```python
from build123d import *

# Parameters (mm, degrees)
F0_W     = 35.3
F0_H     = 35.3
F0_R     = 1.5
F1_DEPTH = 13
F2_R     = 11
F3_DEPTH = 2
F4_R     = 2.25
F5_DEPTH = 24
F7_DEPTH = 3.625
F8_SIZE  = 2.5


with BuildPart() as f1:
    # F0 (on Front) → F1 (new body, symmetric)
    with BuildSketch(Plane.XZ):
        Rectangle(F0_W, F0_H)
        with Locations((-13, -13)):
            Circle(F0_R, mode=Mode.SUBTRACT)
        with Locations((13, -13)):
            Circle(F0_R, mode=Mode.SUBTRACT)
        with Locations((-13, 13)):
            Circle(F0_R, mode=Mode.SUBTRACT)
        with Locations((13, 13)):
            Circle(F0_R, mode=Mode.SUBTRACT)
    extrude(amount=F1_DEPTH, both=True)

    # F2 (on face) → F3 (join)
    with BuildSketch(Plane.XZ.offset(13)):
        Circle(F2_R)
    extrude(amount=F3_DEPTH)

    # F4 (on face) → F5 (join)
    with BuildSketch(Plane.XZ.offset(15)):
        Circle(F4_R)
    extrude(amount=F5_DEPTH)

    # F6 (on Front) → F7 (cut, symmetric)
    with BuildSketch(Plane.XZ):
        Polygon((17.65, 17.65), (11.9931457505, 17.65), (17.65, 11.9931457505), align=None)
        Polygon((11.9931457505, -17.65), (17.65, -17.65), (17.65, -11.9931457505), align=None)
        Polygon((-17.65, -11.9931457505), (-17.65, -17.65), (-11.9931457505, -17.65), align=None)
        Polygon((-11.9931457505, 17.65), (-17.65, 17.65), (-17.65, 11.9931457505), align=None)
    extrude(amount=F7_DEPTH, both=True, mode=Mode.SUBTRACT)

    # F8
    f8_edges = [f1.edges().sort_by_distance(p)[0] for p in [
        (17.65, -8.3125, 17.65),
        (17.65, 8.3125, 17.65),
        (-17.65, 8.3125, 17.65),
        (-17.65, -8.3125, 17.65),
        (17.65, 8.3125, -17.65),
        (17.65, -8.3125, -17.65),
        (-17.65, -8.3125, -17.65),
        (-17.65, 8.3125, -17.65),
    ]]
    chamfer(f8_edges, length=F8_SIZE)


solid = f1.part
```
Source: CAD feature listing. Evaluate the final solid. Frame: model axes, mm. A direction names the side the tool comes from. Give positions to 0.01 mm unless a question says otherwise; leave off trailing zeros. Loops run counter-clockwise (first coordinate to the right, second up) from the corner with the lowest first, then second, coordinate; pieces in that order, holes last. Notation, with made-up numbers: (46, 19) -> (62, 19) arc R21 cw to (62, 23) -> close; hole circle Ø3 at (80, 9). An arc over 180 degrees is marked (long way). Put each result on its own line as item: value. Start each with the question number.
1) Cut plane B-B (x = 13). Return loops of the section in (y, z) (3 decimals), then the cut area to 3 significant figures.
2) Reachability of faces 4 (the face through (-2.38, -13.99, -10.74)), 5 (the face through (-15, 3.625, -15)), 6 (the face through (14.861, 0.051, -14.782)), 7 (the face through (-15, 3.625, 15)) from +Z, -Z, +X, -X, +Y, -Y: full face, straight path, thin tool, end or side. Return the list, or none.
3) Cut plane D-D (x = 0). Return loops of the section in (y, z).
4) Contact query for flat-ended pins moving along their axis: P1, Ø10.5, axis at x = 3, z = -2, coming from the -Y side; P2, Ø5, axis at x = -6.5, y = -31, coming from the +Z side; P3, Ø4.5, axis at x = -15, z = -15.5, coming from the -Y side; P4, Ø1, axis at x = 2.5, y = -18.5, coming from the -Z side. Output: stop coordinate, or through.
5) Material intervals for probe 1 along Z at (x, y) = (-13, -5.25); probe 2 along Z at (x, y) = (-13, -3); probe 3 along Y at (x, z) = (-4.5, -9), sorted ascending.
6) Draft query along X for faces 1 (the face through (0, 0, 17.65)), 2 (the face through (-0.29, -26.83, 2.23)), 3 (the face through (11.5, 0.18, 13.07)). Return one class per face: released by +X, released by -X, zero draft, split by the parting line, or undercut.
7) Cut plane C-C (z = 13). Return loops of the section in (x, y) (3 decimals).
8) Cut plane A-A (y = -7.5). Return loops of the section in (x, z).
Results are:
1. outline: (-13, -17.65) -> (-3.625, -17.65) -> (-3.625, -16.643) -> (3.625, -16.643) -> (3.625, -17.65) -> (13, -17.65) -> (13, -14.5) -> (-13, -14.5) -> close; (-13, -11.5) -> (13, -11.5) -> (13, 11.5) -> (-13, 11.5) -> close; (-13, 14.5) -> (13, 14.5) -> (13, 17.65) -> (3.625, 17.65) -> (3.625, 16.643) -> (-3.625, 16.643) -> (-3.625, 17.65) -> (-13, 17.65) -> close
1. area: 747 mm2
2. face 4: -Y
2. face 5: -Z, -X
2. face 6: -Z, +X
2. face 7: +Z, -X
3. outline: (-39, -2.25) -> (-15, -2.25) -> (-15, -11) -> (-13, -11) -> (-13, -17.65) -> (13, -17.65) -> (13, 17.65) -> (-13, 17.65) -> (-13, 11) -> (-15, 11) -> (-15, 2.25) -> (-39, 2.25) -> close
4. P1: stops at y = -39
4. P2: passes through
4. P3: stops at y = -13
4. P4: stops at z = -1.03
5. probe 1: z = -17.65 to -14.5, -11.5 to 11.5, 14.5 to 17.65
5. probe 2: z = -16.64 to -14.5, -11.5 to 11.5, 14.5 to 16.64
5. probe 3: y = -15 to 13
6. face 1: zero draft
6. face 2: split by the parting line
6. face 3: undercut
7. outline: (-17.65, -13) -> (-14.5, -13) -> (-14.5, 13) -> (-17.65, 13) -> (-17.65, 3.625) -> (-16.643, 3.625) -> (-16.643, -3.625) -> (-17.65, -3.625) -> close; (-11.5, -13) -> (11.5, -13) -> (11.5, 13) -> (-11.5, 13) -> close; (14.5, -13) -> (17.65, -13) -> (17.65, -3.625) -> (16.643, -3.625) -> (16.643, 3.625) -> (17.65, 3.625) -> (17.65, 13) -> (14.5, 13) -> close
8. outline: (-17.65, -15.15) -> (-15.15, -17.65) -> (15.15, -17.65) -> (17.65, -15.15) -> (17.65, 15.15) -> (15.15, 17.65) -> (-15.15, 17.65) -> (-17.65, 15.15) -> close; hole circle Ø3 at (-13, -13); hole circle Ø3 at (-13, 13); hole circle Ø3 at (13, -13); hole circle Ø3 at (13, 13)
